from build123d import *

# Parameters (mm, degrees)
F0_R       = 9
F1_DEPTH   = 26
F3_DEPTH   = 1
F4_R       = 3.5
F7_R       = 2.5
F9_R       = 8
F10_DEPTH  = 25
F13_DEPTH  = 1
F13_FACE_W = 6.5
F13_FACE_H = 1


with BuildPart() as f1:
    # F0 (on Top) → F1 (new body)
    with BuildSketch(Plane.XY):
        Circle(F0_R)
    extrude(amount=F1_DEPTH)



with BuildPart() as f3:
    # F2 (on Right) → F3 (new body, symmetric)
    with BuildSketch(Plane.YZ):
        with BuildLine():
            Line((12.5, 0), (32.5, 0))
            Line((32.5, 0), (32.5, 45))
            ThreePointArc((32.5, 45), (31.0355339059, 48.5355339059), (27.5, 50))
            Line((27.5, 50), (12.5, 50))
            Line((12.5, 50), (12.5, 0))
        make_face()
    extrude(amount=F3_DEPTH, both=True)


with BuildPart() as f1_1:
    add(f1.part)

    add(f3.part)  # F6 merges F3
    # F6: sweep along a path in F5
    with BuildLine(Plane.YZ) as f6_path:
        Line((-20, 0), (0, 0))
        Line((0, 0), (15, 0))
        ThreePointArc((15, 0), (18.5355339059, 1.4644660941), (20, 5))
        Line((20, 5), (20, 50))
    # F4 (on Front) → F6 (sweep)
    with BuildSketch(Plane.XZ):
        Circle(F4_R)
    sweep(path=f6_path.line)

    # F8: sweep along a path in F5
    with BuildLine(Plane.YZ) as f8_path:
        Line((-20, 0), (0, 0))
        Line((0, 0), (15, 0))
        ThreePointArc((15, 0), (18.5355339059, 1.4644660941), (20, 5))
        Line((20, 5), (20, 50))
    # F7 (on face) → F8 (sweep, cut)
    with BuildSketch(Plane.XZ.offset(20)):
        Circle(F7_R)
    sweep(path=f8_path.line, mode=Mode.SUBTRACT)

    # F9 (on face) → F10 (cut)
    with BuildSketch(Plane.XY.offset(26)):
        Circle(F9_R)
    extrude(amount=-F10_DEPTH, mode=Mode.SUBTRACT)

    # F12 (on face) → F13 (join)
    with BuildSketch(Plane.XY.offset(50)):
        with BuildLine():
            Line((7.5, 25), (1, 25))
            Line((1, 25), (1, 23.3541019662))
            ThreePointArc((1, 23.3541019662), (3.5, 20), (1, 16.6458980338))
            Line((1, 16.6458980338), (1, 12.5))
            Line((1, 12.5), (2.5, 12.5))
            ThreePointArc((2.5, 12.5), (6.0355339059, 13.9644660941), (7.5, 17.5))
            Line((7.5, 17.5), (7.5, 25))
        make_face()
        with BuildLine():
            Line((-1, 25), (-7.5, 25))
            Line((-7.5, 25), (-7.5, 17.5))
            ThreePointArc((-7.5, 17.5), (-6.0355339059, 13.9644660941), (-2.5, 12.5))
            Line((-2.5, 12.5), (-1, 12.5))
            Line((-1, 12.5), (-1, 16.6458980338))
            ThreePointArc((-1, 16.6458980338), (-3.5, 20), (-1, 23.3541019662))
            Line((-1, 23.3541019662), (-1, 25))
        make_face()
    extrude(amount=-F13_DEPTH)

    # F14: sweep along a path in F14_path
    with BuildLine(Plane(origin=(1, 27.5, 50), x_dir=(0, 0, 1), z_dir=(1, 0, 0))) as f14_path:
        Line((0, 2.5), (0, 0))
        ThreePointArc((0, 0), (-1.4644660941, -3.5355339059), (-5, -5))
        Line((-5, -5), (-50, -5))
    # F13_face (on face) → F14 (sweep)
    with BuildSketch(Plane(origin=(4.25, 25, 49.5), x_dir=(-1, 0, 0), z_dir=(0, 1, 0))):
        Rectangle(F13_FACE_W, F13_FACE_H)
        with Locations((8.5, 0)):
            Rectangle(F13_FACE_W, F13_FACE_H)
    sweep(path=f14_path.line)


solid = f1_1.part
Part model, mm, in its own coordinate system. A direction names the side the tool comes from. Round coordinates to 2 decimals unless told otherwise and drop trailing zeros. Order: outer loops, then holes, each group sorted by start corner. A loop starts at its lowest first (then second) coordinate and runs counter-clockwise, first axis right, second up. Notation, with made-up numbers: (86.25, 52) -> (141.25, 52) arc R26 cw to (141.25, 87) -> close; hole circle Ø8 at (76, 68.25). An arc over 180 degrees is marked (long way). Put each result on its own line as item: value.
Q1. Tool access for faces 4 (the face through (-4, 20, 49)), 5 (the face through (4.204, 30.297, 47.859)), 6 (the face through (7.5, 32, 33)), 7 (the face through (-0.33, 22.48, 27.82)): list every direction of +Z, -Z, +X, -X, +Y, -Y with a clear straight run to the whole face (end or side of a thin tool).
From the geometry:
face 4: -X
face 5: -Z, +X
face 6: +Z, -Z, +X, +Y
face 7: +Z
Q2. Band-saw the part on B-B (z = 40). Give the cut face in (x, y).
From the geometry:
outline: (-7.5, 31.5) -> (-1, 31.5) -> (-1, 23.35) arc R3.5 ccw to (-1, 16.65) -> (-1, 12.5) -> (1, 12.5) -> (1, 16.65) arc R3.5 ccw to (1, 23.35) -> (1, 31.5) -> (7.5, 31.5) -> (7.5, 32.5) -> (-7.5, 32.5) -> close; hole circle Ø5 at (0, 20)
Q3. Band-saw the part on D-D (y = 24). Give the cut face in (x, z), and give its area (3 significant figures).
From the geometry:
outline: (-7.5, 49) -> (-1, 49) -> (-1, 0) -> (1, 0) -> (1, 49) -> (7.5, 49) -> (7.5, 50) -> (-7.5, 50) -> close
area: 113 mm2
Q4. Band-saw the part on C-C (x = -4.75). Give the cut face in (y, z).
From the geometry:
outline: (-7.64, 0) -> (7.64, 0) -> (7.64, 26) -> (6.44, 26) -> (6.44, 1) -> (-6.44, 1) -> (-6.44, 26) -> (-7.64, 26) -> close; (13.03, 49) -> (27.5, 49) arc R4 cw to (31.5, 45) -> (31.5, 0) -> (32.5, 0) -> (32.5, 45) arc R5 ccw to (27.5, 50) -> (13.03, 50) -> close
Q5. Wall check: line 1 (Y direction, x = 0, z = 15.5); line 2 (Y direction, x = -0.5, z = 8.5); line 3 (Y direction, x = -0.25, z = 32). Give the ranges that are in metal, low to high. Write a range as [from, to].
From the geometry:
line 1: y = [-9, -8], [8, 9], [12.5, 17.5], [22.5, 32.5]
line 2: y = [-8.99, -7.98], [7.98, 8.99], [12.5, 17.55], [22.45, 32.5]
line 3: y = [12.5, 17.51], [22.49, 32.5]
Q6. Pull direction X, two halves, no side cores. Call faces 1 (the face through (4, 0, 1)), 2 (the face through (1, 15, 26)), 3 (the face through (-4.296, 30.297, 47.859)): pulls with the +X half, pulls with the -X half, needs draft (parallel to the pull), parting line crosses it, or undercut.
From the geometry:
face 1: undercut
face 2: pulls with the +X half
face 3: needs draft
Q7. Pin check, flat tips, straight feed: pin 1 Ø2 at (y, z) = (14, 23) entering from -X; pin 2 Ø4 at (x, y) = (-4.5, 3.5) entering from -Z; pin 3 Ø11 at (y, z) = (28, 21.5) entering from +X. Stop position of each tip, or through.
From the geometry:
pin 1: stops at x = -1
pin 2: stops at z = -2.45
pin 3: stops at x = 7.5
Q8. Band-saw the part on A-A (z = 10). Give the cut face in (x, y), and give its area (3 significant figures).
From the geometry:
outline: circle Ø18 at (0, 0); (-7.5, 31.5) -> (-1, 31.5) -> (-1, 23.35) arc R3.5 ccw to (-1, 16.65) -> (-1, 12.5) -> (1, 12.5) -> (1, 16.65) arc R3.5 ccw to (1, 23.35) -> (1, 31.5) -> (7.5, 31.5) -> (7.5, 32.5) -> (-7.5, 32.5) -> close; hole circle Ø16 at (0, 0); hole circle Ø5 at (0, 20)
area: 111 mm2
